Input: dimensioned drawing with shaded views. Units: mm. Origin: part minimum x, y, z. Give positions to 0.01 mm unless a question says otherwise; leave off trailing zeros. Order: outer loops, then holes, each group sorted by start corner. A loop starts at its lowest first (then second) coordinate and runs counter-clockwise, first axis right, second up. Notation, with made-up numbers: (80, 23.5) -> (98, 23.5) arc R22 cw to (98, 57.5) -> close; hole circle Ø8 at (-22, 83). An arc over 180 degrees is marked (long way). One line per question, with ' | ' between items. Start each with the question number.
(1) Section C-C (z = 69). Return loops of the section in (x, y).
(2) Section A-A (z = 84). Return loops of the section in (x, y).
(3) Ray query, L1, parallel to X at y = 2.5, z = 27.5; L2, parallel to Z at x = 22, y = 2.1; L3, parallel to Y at x = 116, z = 44. Return the intervals inside material, ascending.
(4) Section B-B (x = 102.5). Return loops of the section in (y, z), then the cut area to 3 significant figures.
(5) Mould query, pull axis Z, two halves, no side actions, for the marked faces 1 and 2. Classes: +Z half, -Z half, draft (parallel to the pull), parting line (faces both ways), or undercut.
(6) Section D-D (x = 71). Return loops of the section in (y, z).
(7) First-contact query: pin 1 Ø0.5 at (x, y) = (101.5, 2.5) entering from -Z; pin 2 Ø1 at (x, y) = (65.5, 1) entering from -Z; pin 3 Ø1.1 at (x, y) = (22.5, 2.5) entering from +Z. Flat tips, straight axial feed; report the tip coordinate or a pass-through.
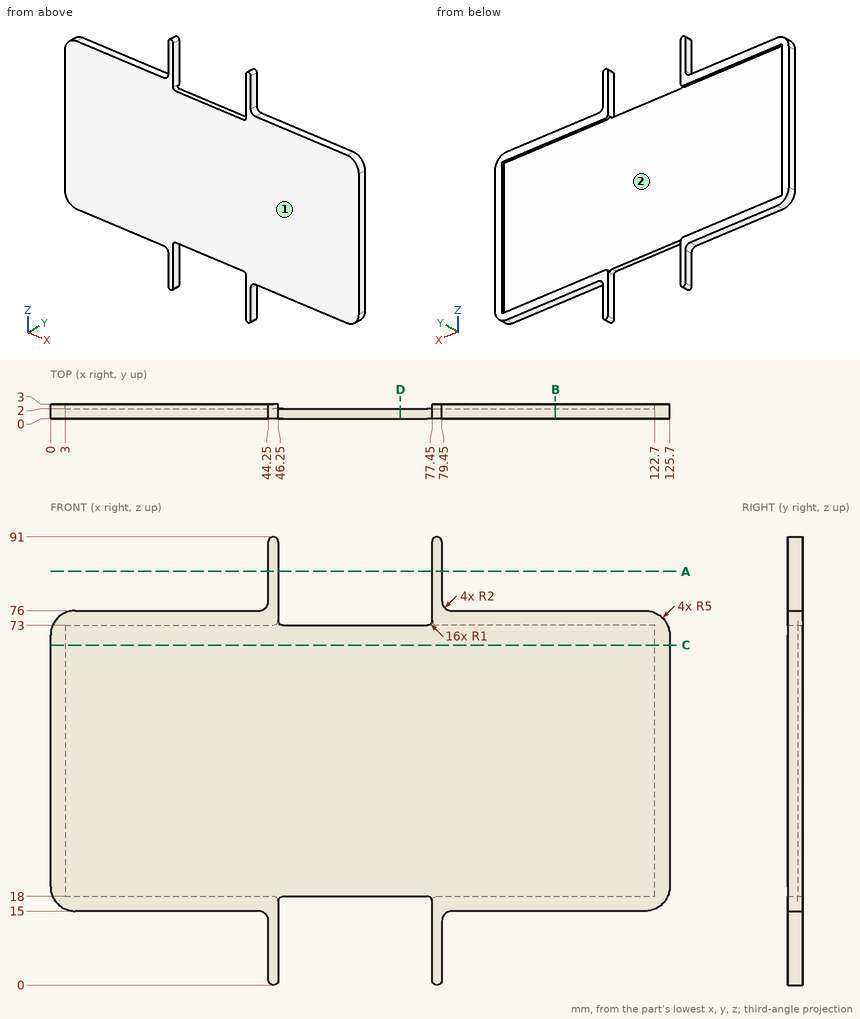
Response:
1) outline: (0, 0) -> (125.7, 0) -> (125.7, 3) -> (122.7, 3) -> (122.7, 2) -> (3, 2) -> (3, 3) -> (0, 3) -> close
2) outline: (44.25, 0) -> (46.25, 0) -> (46.25, 3) -> (44.25, 3) -> close; (77.45, 0) -> (79.45, 0) -> (79.45, 3) -> (77.45, 3) -> close
3) L1: x = 0 to 3, 122.7 to 125.7 | L2: z = 15 to 18, 73 to 76 | L3: y = 0 to 2
4) outline: (0, 15) -> (3, 15) -> (3, 18) -> (2, 18) -> (2, 73) -> (3, 73) -> (3, 76) -> (0, 76) -> close | area: 128 mm^2
5) face 1: draft | face 2: undercut
6) outline: (0, 18) -> (2, 18) -> (2, 73) -> (0, 73) -> close
7) pin 1: stops at z = 15 | pin 2: stops at z = 18 | pin 3: stops at z = 76
